The model under review builds one solid part; all positions refer to its coordinate system, in mm. Give positions to 0.01 mm unless a question says otherwise; leave off trailing zeros. Write each loop counter-clockwise with the first axis right and the second up, starting at its lowest first coordinate (ties: lowest second). Pieces come first, ordered by that corner, then holes. Notation, with made-up numbers: (25, 59) -> (30, 59) arc R23 ccw to (30, 82) -> close; hole circle Ø8 at (57.5, 79). An arc over 180 degrees is marked (long way). Use CSV: the item, a comma, the result in double quotes.
Autodesk Inventor part; units mm, degrees
ref_plane "YZ Plane" through (0, 0, 0) normal (1, 0, 0) x (0, 1, 0)
ref_plane "XZ Plane" through (0, 0, 0) normal (0, 1, 0) x (-1, 0, 0)
ref_plane "XY Plane" through (0, 0, 0) normal (0, 0, 1) x (1, 0, 0)
sketch "Sketch2" plane through (0, 0, 0) normal (0, 1, 0) x (-1, 0, 0)
  line L0 (-89, 99) -> (89, 99)
  line L1 (89, 99) -> (89, -99)
  line L2 (89, -99) -> (-89, -99)
  line L3 (-89, -99) -> (-89, 99)
  line L4 (-89, 99) -> (89, -99) construction
  line L5 (89, 99) -> (-89, -99) construction
  line L6 (-89, 99) -> (89, 99)
  line L7 (89, 99) -> (89, -81)
  line L8 (89, -81) -> (-89, -81)
  line L9 (-89, -81) -> (-89, 99)
  line L10 (-4.5, 99) -> (-89, 99)
  line L11 (-89, 99) -> (-89, 43)
  line L12 (-89, 43) -> (-4.5, 43)
  line L13 (-4.5, 43) -> (-4.5, 99)
  line L14 (4.5, 99) -> (89, 99)
  line L15 (89, 99) -> (89, 43)
  line L16 (89, 43) -> (4.5, 43)
  line L17 (4.5, 43) -> (4.5, 99)
  line L18 (22.5, 77.5) -> (22.5, 66.5)
  line L19 (16.5, 66.5) -> (16.5, 77.5)
  line L20 (-22.5, 66.5) -> (-22.5, 77.5)
  line L21 (-16.5, 77.5) -> (-16.5, 66.5)
  line L22 (-23.5, 99) -> (-16.5, 99)
  line L23 (-16.5, 99) -> (-16.5, 43)
  line L24 (-16.5, 43) -> (-23.5, 43)
  line L25 (-23.5, 43) -> (-23.5, 99)
  line L26 (16.5, 99) -> (23.5, 99)
  line L27 (23.5, 99) -> (23.5, 43)
  line L28 (23.5, 43) -> (16.5, 43)
  line L29 (16.5, 43) -> (16.5, 99)
  line L30 (-89, 99) -> (89, 99)
  line L31 (89, 99) -> (89, 98)
  line L32 (89, 98) -> (-89, 98)
  line L33 (-89, 98) -> (-89, 99)
  line L34 (89, -81) -> (74, -81)
  line L35 (74, -81) -> (74, -61)
  line L36 (74, -61) -> (89, -61)
  line L37 (89, -61) -> (89, -81)
  line L38 (-89, -81) -> (-74, -81)
  line L39 (-74, -81) -> (-74, -61)
  line L40 (-74, -61) -> (-89, -61)
  line L41 (-89, -61) -> (-89, -81)
  line L42 (16.5, 98) -> (-16.5, 98)
  line L43 (-16.5, 98) -> (-16.5, 94)
  line L44 (-16.5, 94) -> (16.5, 94)
  line L45 (16.5, 94) -> (16.5, 98)
  line L46 (-84.4, -75) -> (-84.4, -71.5)
  line L47 (-84.4, -71.5) -> (-87, -71.5)
  line L48 (-87, -71.5) -> (-87, -75)
  line L49 (-87, -75) -> (-84.4, -75)
  line L50 (-79.6, -75) -> (-77, -75)
  line L51 (-77, -75) -> (-77, -71.5)
  line L52 (-77, -71.5) -> (-79.6, -71.5)
  line L53 (-79.6, -71.5) -> (-79.6, -75)
  line L54 (-75, -78) -> (-89, -78)
  line L55 (-89, -78) -> (-89, -63)
  line L56 (-89, -63) -> (-75, -63)
  line L57 (-75, -63) -> (-75, -78)
  circle A0 centre (-80.45, -67.25) radius 1.25
  point P0 (0, 0)
  point P1 (4.5, 99)
  point P2 (-4.5, 99)
  point P3 (-89, 43)
  point P4 (89, 43)
  point P5 (4.5, 98)
  point P6 (-4.5, 98)
  point P7 (-16.5, 98)
  point P8 (-23.5, 98)
  point P9 (23.5, 98)
  point P10 (16.5, 98)
  point P11 (-4.5, 94)
  point P12 (4.5, 94)
  point P13 (16.5, 94)
  dimension "d8" = 178
  dimension "d9" = 198
  dimension "d10" = 18
  dimension "d11" = 84.5
  dimension "d13" = 84.5
  dimension "d17" = 9
  dimension "d18" = 1
  dimension "d19" = 15
  dimension "d20" = 20
  dimension "d21" = 15
  dimension "d22" = 20
  dimension "d75" = 55
  dimension "d76" = 55
  dimension "d77" = 7
  dimension "d78" = 7
  dimension "d79" = 4
extrude "Extrusion2" add sketch "Sketch2" along normal blind 3 contours L32 L23 L21 L12 L25 | L12 L13 L44 L17 L16 L1 L36 L35 L8 L39 L40 L3 | L32 L13 L44 L23 | L32 L17 L44 L13 | L32 L29 L44 L17 | L32 L27 L16 L29 L19
fillet "Fillet1" radius 3 6 edges at (23.5, 1.5, 43) (-23.5, 1.5, 43) (-16.5, 1.5, 43) (-4.5, 1.5, 43) (4.5, 1.5, 43) (16.5, 1.5, 43)
fillet "Fillet2" radius 3 2 edges at (74, 1.5, -61) (-74, 1.5, -61)
fillet "Fillet3" radius 3 4 edges at (16.5, 1.5, 94) (4.5, 1.5, 94) (-4.5, 1.5, 94) (-16.5, 1.5, 94)
equation "\"d11\" = d13"
properties part number "base" material "Aluminum 6061"
Q1. Insertion check: pin 1 (0.9 mm diameter, centred on x = 86, y = 1.5, fed in from -Z); pin 2 (1.5 mm diameter, centred on y = 1, z = 74.5, fed in from +X); pin 3 (1.5 mm diameter, centred on y = 1.5, z = 58, fed in from -X). Each pin has a flat end and moves straight along its axis. Give the tip position at first contact, or say it passes through.
Derived:
pin 1,"stops at z = -61"
pin 2,"stops at x = 23.5"
pin 3,"stops at x = -23.5"
Q2. Consider section C-C (x = 54). Write out the cut boundary in (y, z), then the cut area to 3 significant figures.
Derived:
outline,"(0, -81) -> (3, -81) -> (3, 43) -> (0, 43) -> close"
area,"372 mm2"
Q3. To check wall thickness, follow probe 1 along X at (y, z) = (1.35, 70); probe 2 along Z at (x, y) = (-9, 0.5); probe 3 along Z at (x, y) = (-71, 1.9). State the ranges of each line that lie inside material, in increasing order.
Derived:
probe 1,"x = -23.5 to -16.5, -4.5 to 4.5, 16.5 to 23.5"
probe 2,"z = -81 to 43, 94 to 98"
probe 3,"z = -81 to 43"
Q4. Consider section A-A (z = 50.5). Write out the cut boundary in (x, y).
Derived:
outline,"(-23.5, 0) -> (-16.5, 0) -> (-16.5, 3) -> (-23.5, 3) -> close; (-4.5, 0) -> (4.5, 0) -> (4.5, 3) -> (-4.5, 3) -> close; (16.5, 0) -> (23.5, 0) -> (23.5, 3) -> (16.5, 3) -> close"
Q5. Consider section B-B (y = 1.95). State how many separate pieces and enclosed holes the cut face has, then the cut area to 3 significant figures.
Derived:
separate pieces,"1"
enclosed holes,"2"
area,"22,900 mm2"
